For this review, take the finished solid that the model builds, in its own axes (mm). Face numbers are marked on the shaded views. A direction names the side the tool comes from. Give positions to 0.01 mm unless a question says otherwise; leave off trailing zeros. Loops run counter-clockwise (first coordinate to the right, second up) from the corner with the lowest first, then second, coordinate; pieces in that order, holes last.
Autodesk Inventor part; units mm, degrees
ref_plane "YZ Plane" through (0, 0, 0) normal (1, 0, 0) x (0, 1, 0)
ref_plane "XZ Plane" through (0, 0, 0) normal (0, 1, 0) x (-1, 0, 0)
ref_plane "XY Plane" through (0, 0, 0) normal (0, 0, 1) x (1, 0, 0)
sketch "Sketch1" plane through (0, 0, 0) normal (0, 0, 1) x (1, 0, 0)
  line L0 (0, 23.3816) -> (34.8458, 23.3816)
  line L1 (36.8458, 21.3816) -> (36.8458, 2)
  line L2 (38.8458, 0) -> (55.1987, 0)
  line L3 (55.1987, 0) -> (55.1987, 6)
  line L4 (55.1987, 6) -> (44.8458, 6)
  line L5 (42.8458, 8) -> (42.8458, 27.3816)
  line L6 (40.8458, 29.3816) -> (0, 29.3816)
  arc A0 (42.8458, 8) -> (44.8458, 6) centre (44.8458, 8) ccw
  arc A1 (36.8458, 2) -> (38.8458, 0) centre (38.8458, 2) ccw
  arc A2 (36.8458, 21.3816) -> (34.8458, 23.3816) centre (34.8458, 21.3816) ccw
  arc A3 (42.8458, 27.3816) -> (40.8458, 29.3816) centre (40.8458, 27.3816) ccw
  line L7 (0, 23.3816) -> (0, 29.3816)
  point P0 (0, 0)
  dimension "d0" = 6
  dimension "d1" = 6
  dimension "d2" = 6
  dimension "d3" = 2
extrude "Extrusion1" add sketch "Sketch1" along normal blind 20
sketch "Sketch2" plane through (44.8458, 6, 0) normal (0, 1, 0) x (1, 0, 0)
  line L0 (10.3529, -20) -> (0, -20) construction
  line L1 (5.1765, -20) -> (5.1765, -15) construction
  line L2 (5.1765, -15) -> (5.1765, -5) construction
  circle A0 centre (5.1765, -15) radius 2
  circle A1 centre (5.1765, -5) radius 2
  point P0 (-44.8458, 0)
  dimension "d7" = 10
  dimension "d8" = 5
  dimension "d9" = 4
  dimension "d10" = 4
extrude "Extrusion2" cut sketch "Sketch2" against normal blind 20
mirror "Mirror1" about plane through (0, 29.3816, 0) normal (-1, 0, 0) of "Extrusion1", "Extrusion2"
properties part number "poigne"
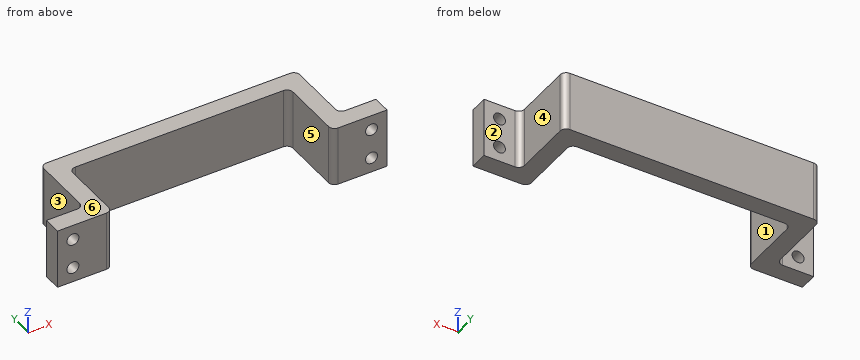
Item 1: For L1, parallel to X at y = 3.7, z = 5; L2, parallel to X at y = 1.7, z = 15; L3, parallel to X at y = 8.5, z = 7, list the stretches that pass through material, from the lowest coordinate up.
Answer:
L1: x = -55.2 to -52.02, -48.02 to -36.85, 36.85 to 48.02, 52.02 to 55.2
L2: x = -55.2 to -52.02, -48.02 to -36.87, 36.87 to 48.02, 52.02 to 55.2
L3: x = -42.85 to -36.85, 36.85 to 42.85
Item 2: Tool access review of the marked faces 1, 2 and 3: name each direction out of +Z, -Z, +X, -X, +Y, -Y from which nothing blocks a thin tool from reaching the whole face with its end or side.
Answer:
face 1: +Z, -Z, -Y
face 2: +Z, -Z, +X, +Y
face 3: +Z, -Z, -X, +Y
Item 3: Take a section at B-B on y = 9.25. Give the boundary of the cut face in (x, z).
Answer:
outline: (-42.85, 0) - (-36.85, 0) - (-36.85, 20) - (-42.85, 20) - close; (36.85, 0) - (42.85, 0) - (42.85, 20) - (36.85, 20) - close
Item 4: The part is to be moulded in two halves that separate along X. For the marked faces 4, 5 and 6, say which applies: released by +X, released by -X, zero draft, split by the parting line, or undercut.
Answer:
face 4: released by +X
face 5: undercut
face 6: zero draft
Item 5: Take a section at D-D on x = 12. Give the boundary of the cut face in (y, z), and give its area (3 significant figures).
Answer:
outline: (23.38, 0) - (29.38, 0) - (29.38, 20) - (23.38, 20) - close
area: 120 mm2
Item 6: Take a section at A-A on z = 15. Give the boundary of the cut face in (x, y).
Answer:
outline: (-55.2, 0) - (-52.02, 0) - (-52.02, 6) - (-55.2, 6) - close; (-48.02, 0) - (-38.85, 0) arc R2 ccw to (-36.85, 2) - (-36.85, 21.38) arc R2 cw to (-34.85, 23.38) - (34.85, 23.38) arc R2 cw to (36.85, 21.38) - (36.85, 2) arc R2 ccw to (38.85, 0) - (48.02, 0) - (48.02, 6) - (44.85, 6) arc R2 cw to (42.85, 8) - (42.85, 27.38) arc R2 ccw to (40.85, 29.38) - (-40.85, 29.38) arc R2 ccw to (-42.85, 27.38) - (-42.85, 8) arc R2 cw to (-44.85, 6) - (-48.02, 6) - close; (52.02, 0) - (55.2, 0) - (55.2, 6) - (52.02, 6) - close
Item 7: Clearance check with flat-ended pins moving along their axes: pin 1 Ø10 at (x, z) = (10.5, 11) entering from -Y; pin 2 Ø3 at (x, z) = (-50.02, 5) entering from -Y; pin 3 Ø1 at (y, z) = (18, 6.5) entering from +X; pin 4 Ø5 at (x, z) = (-48, 12) entering from +Y. State where each tip first meets the part, or that it passes through.
Answer:
pin 1: stops at y = 23.38
pin 2: passes through
pin 3: stops at x = 42.85
pin 4: stops at y = 6
Item 8: Take a section at C-C on z = 8.5. Give the boundary of the cut face in (x, y).
Answer:
outline: (-55.2, 0) - (-38.85, 0) arc R2 ccw to (-36.85, 2) - (-36.85, 21.38) arc R2 cw to (-34.85, 23.38) - (34.85, 23.38) arc R2 cw to (36.85, 21.38) - (36.85, 2) arc R2 ccw to (38.85, 0) - (55.2, 0) - (55.2, 6) - (44.85, 6) arc R2 cw to (42.85, 8) - (42.85, 27.38) arc R2 ccw to (40.85, 29.38) - (-40.85, 29.38) arc R2 ccw to (-42.85, 27.38) - (-42.85, 8) arc R2 cw to (-44.85, 6) - (-55.2, 6) - close
